Here's how the part is built. I have some questions about the finished solid (model axes, mm). Face numbers are marked on the shaded views. A direction names the side the tool comes from. Coordinates: 2 decimals unless noted, no trailing zeros. Loops run counter-clockwise (first coordinate to the right, second up) from the corner with the lowest first, then second, coordinate; pieces in that order, holes last. Notation, with made-up numbers: (43, 19) - (65, 19) arc R23 cw to (65, 49) - close; hole circle Ø5 at (12, 69.5). An arc over 180 degrees is marked (long way). Use a Markdown table: item, result.
```python
from build123d import *

# Parameters (mm, degrees)
MODEL_R                 = 1.25
BOSS_EXTRUDE1_DEPTH     = 2
BOSS_EXTRUDE2_DEPTH     = 11.50072
SKETCH2_R               = 1.25
CUT_EXTRUDE1_DEPTH      = 2
CUT_EXTRUDE1_DEPTH_BACK = 4
SKETCH3_W               = 9.00072
SKETCH3_H               = 2
SKETCH3_W_2             = 8.20072
SKETCH3_H_2             = 1.2
CUT_EXTRUDE2_DEPTH      = 4


with BuildPart() as part:
    # Model → Boss-Extrude1 (new body)
    with BuildSketch(Plane.XY):
        Polygon((1.25, 4), (0, 4), (0, 8), (1.25, 8), (1.25, 12), (10.25072, 12), (10.25072, 8), (11.50072, 8), (11.50072, 4), (10.25072, 4), (10.25072, 0), (1.25, 0), align=None)
        with Locations((7.75072, 6)):
            Circle(MODEL_R, mode=Mode.SUBTRACT)
        with Locations((3.75, 6)):
            Circle(MODEL_R, mode=Mode.SUBTRACT)
    extrude(amount=BOSS_EXTRUDE1_DEPTH)

    # Sketch1 → Boss-Extrude2 (add)
    with BuildSketch(Plane.ZY):
        with BuildLine():
            Line((2, 4), (2, 5))
            ThreePointArc((2, 5), (2.292893219, 4.292893219), (3, 4))
            Line((3, 4), (2, 4))
        make_face()
        with BuildLine():
            Line((0, 4), (-1, 4))
            ThreePointArc((-1, 4), (-0.292893219, 4.292893219), (0, 5))
            Line((0, 5), (0, 4))
        make_face()
    extrude(amount=-BOSS_EXTRUDE2_DEPTH)

    # Sketch2 → Cut-Extrude1 (cut, two sides)
    with BuildSketch(Plane.XY.offset(2)) as cut_extrude1_sk:
        with Locations((3.75, 6)):
            Circle(SKETCH2_R)
        with Locations((7.75072, 6)):
            Circle(SKETCH2_R)
    extrude(amount=CUT_EXTRUDE1_DEPTH, mode=Mode.SUBTRACT)
    extrude(cut_extrude1_sk.sketch, amount=-CUT_EXTRUDE1_DEPTH_BACK, mode=Mode.SUBTRACT)

    # Sketch3 → Cut-Extrude2 (cut)
    with BuildSketch(Plane(origin=(0, 12, 0), x_dir=(1, 0, 0), z_dir=(0, 1, 0))):
        with Locations((5.75036, -1)):
            Rectangle(SKETCH3_W, SKETCH3_H)
        with Locations((5.75036, -1)):
            Rectangle(SKETCH3_W_2, SKETCH3_H_2, mode=Mode.SUBTRACT)
    extrude(amount=-CUT_EXTRUDE2_DEPTH, mode=Mode.SUBTRACT)


solid = part.part
```
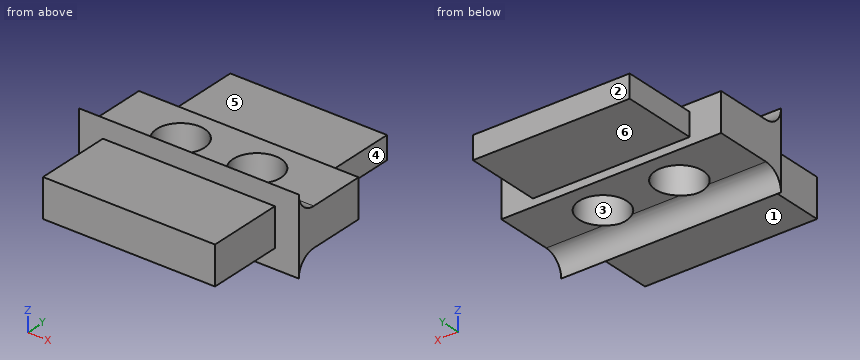
Q1. I want a section at C-C, the plane x = 3.75. Write out the boundary of the cut face in (y, z), then the cut area to 3 significant figures.
Check values:
| item | result |
|---|---|
| outline | (0, 0) - (4, 0) - (4, -1) arc R1 cw to (4.75, -0.03) - (4.75, 2.03) arc R1 cw to (4, 3) - (4, 2) - (0, 2) - close; (7.25, 0) - (8, 0) - (8, 0.4) - (12, 0.4) - (12, 1.6) - (8, 1.6) - (8, 2) - (7.25, 2) - close |
| area | 16.2 mm^2 |
Q2. If we mould it in two halves opening along Y, with no side actions, what happens to the marked faces 1, 2 and 3? For each: pulls with the +Y half, pulls with the -Y half, needs draft (parallel to the pull), parting line crosses it, or undercut.
Check values:
| item | result |
|---|---|
| face 1 | needs draft |
| face 2 | pulls with the +Y half |
| face 3 | undercut |
Q3. I want a section at D-D, the plane x = 11. Write out the boundary of the cut face in (y, z), then the cut area to 3 significant figures.
Check values:
| item | result |
|---|---|
| outline | (4, -1) arc R1 cw to (5, 0) - (8, 0) - (8, 2) - (5, 2) arc R1 cw to (4, 3) - close |
| area | 8.43 mm^2 |
Q4. Will these pins go through, and if not, where does the flat tip stop? P1, Ø2, axis at x = 8, y = 2, coming from the -Z side; P2, Ø2, axis at x = 6, y = 9.5, coming from the -Z side; P3, Ø1, axis at y = 2, z = 1, coming from the -X side.
Check values:
| item | result |
|---|---|
| P1 | z = 0 |
| P2 | z = 0.4 |
| P3 | x = 1.25 |
Q5. Which directions (+Z, -Z, +X, -X, +Y, -Y) give clear straight access to the entire face, cutting with the end or side of a thin tool? Please do the marked faces 4, 5 and 6.
Check values:
| item | result |
|---|---|
| face 4 | +Z, -Z, +X, +Y |
| face 5 | +Z, +X, -X, +Y |
| face 6 | -Z, +X, -X, +Y |
Q6. I want a section at B-B, the plane z = 1. Write out the boundary of the cut face in (x, y).
Check values:
| item | result |
|---|---|
| outline | (0, 4) - (1.25, 4) - (1.25, 0) - (10.25, 0) - (10.25, 4) - (11.5, 4) - (11.5, 8) - (9.85, 8) - (9.85, 12) - (1.65, 12) - (1.65, 8) - (0, 8) - close; hole circle Ø2.5 at (3.75, 6); hole circle Ø2.5 at (7.75, 6) |
Q7. Please list where these lines run through material, in increasing order: L1, parallel to X at y = 6, z = 0.95; L2, parallel to Y at x = 3.75, z = 1.5; L3, parallel to X at y = 6.5, z = 0.05. Write a range as from..to.
Check values:
| item | result |
|---|---|
| L1 | 0..2.5, 5..6.5, 9..11.5 |
| L2 | 0..4.75, 7.25..12 |
| L3 | 0..2.6, 4.9..6.61, 8.9..11.5 |
Q8. I want a section at A-A, the plane y = 6. Write out the boundary of the cut face in (x, z), then the cut area to 3 significant figures.
Check values:
| item | result |
|---|---|
| outline | (0, 0) - (2.5, 0) - (2.5, 2) - (0, 2) - close; (5, 0) - (6.5, 0) - (6.5, 2) - (5, 2) - close; (9, 0) - (11.5, 0) - (11.5, 2) - (9, 2) - close |
| area | 13.0 mm^2 |
